from build123d import *

# Parameters (mm, degrees)
SKETCH2_R           = 1.5
BOSS_EXTRUDE1_DEPTH = 5


with BuildPart() as part:
    # Sketch2 → Boss-Extrude1 (new body)
    with BuildSketch(Plane.XY):
        with BuildLine():
            Line((2.043003371, 9.789082553), (85.846562924, -7.700907316))
            Line((85.846562924, -7.700907316), (81.760556182, -27.279072422))
            Line((81.760556182, -27.279072422), (-2.043003371, -9.789082553))
            ThreePointArc((-2.043003371, -9.789082553), (-9.789082553, 2.043003371), (2.043003371, 9.789082553))
        make_face()
        Circle(SKETCH2_R, mode=Mode.SUBTRACT)
        with Locations((0, 7)):
            Circle(SKETCH2_R, mode=Mode.SUBTRACT)
        with Locations((0, -7)):
            Circle(SKETCH2_R, mode=Mode.SUBTRACT)
        with Locations((7, 0)):
            Circle(SKETCH2_R, mode=Mode.SUBTRACT)
        with Locations((-7, 0)):
            Circle(SKETCH2_R, mode=Mode.SUBTRACT)
        Polygon((74.456281443, -8.470092426), (67.882907111, -10.632764358), (66.469148778, -17.406809485), (71.628764778, -22.018182679), (78.20213911, -19.855510747), (79.615897443, -13.08146562), align=None, mode=Mode.SUBTRACT)
    extrude(amount=BOSS_EXTRUDE1_DEPTH)


solid = part.part
Design review of the part built by this model. Coordinates are the model's own, in mm. A direction names the side the tool comes from. Round coordinates to 2 decimals unless told otherwise and drop trailing zeros. Loops run counter-clockwise (first coordinate to the right, second up) from the corner with the lowest first, then second, coordinate; pieces in that order, holes last. Notation, with made-up numbers: (88.25, -7) - (111.25, -7) arc R21 cw to (111.25, 17) - close; hole circle Ø10 at (-19.5, -17). An arc over 180 degrees is marked (long way). One line per item, written item: value. Start each with the question number.
1) Consider section A-A on z = 1.55. Give the boundary of the cut face in (x, y).
2) Draft analysis for pull direction Y (two halves, no side actions). For faces 3 (the cylindrical face through (-0.325, -8.464, 2.465)), 4 (the flat face through (43.358, 1.167, 2.465)), 5 (the flat face through (69.01, -19.68, 2.46)), 6 (the cylindrical face through (-9.83, 1.83, 2.46)), state which applies: +Y half, -Y half, draft (parallel to the pull), parting line (faces both ways), or undercut.
3) Consider section C-C on x = 73.5. Give the boundary of the cut face in (y, z).
4) To check wall thickness, follow L1, parallel to Y at x = 0, z = 3.9; L2, parallel to Y at x = 7, z = 2.15; L3, parallel to Y at x = 77.5, z = 1.5. State the ranges of each line that lie inside material, in increasing order. Write a range as from..to.
5) Consider section B-B on y = 0. Give the boundary of the cut face in (x, z).
6) Consider section D-D on y = -21. Give the boundary of the cut face in (x, z).
7) Insertion check: pin 1 Ø12 at (x, y) = (27, -11) entering from -Z; pin 2 Ø1.5 at (y, z) = (-15.5, 1) entering from +X; pin 3 Ø1.5 at (y, z) = (-10, 3) entering from -X; pin 4 Ø1 at (y, z) = (-17.5, 1.5) entering from +X. Each pin has a flat end and moves straight along its axis. Give the tip position at first contact, or say it passes through.
8) For faces 1 (the flat face through (67.186, -13.972, 2.465)), 2 (the flat face through (39, -8, 0)), list the 3-axis set-ups (+Z, -Z, +X, -X, +Y, -Y) from which the entire face can be reached by the end or side of a thin tool; tool diameter is ignored.
Reported:
1. outline: (-2.04, -9.79) - (81.76, -27.28) - (85.85, -7.7) - (2.04, 9.79) arc R10 ccw to start; hole circle Ø3 at (-7, 0); hole circle Ø3 at (0, -7); hole circle Ø3 at (0, 0); hole circle Ø3 at (0, 7); hole circle Ø3 at (7, 0); hole (66.47, -17.41) - (71.63, -22.02) - (78.2, -19.86) - (79.62, -13.08) - (74.46, -8.47) - (67.88, -10.63) - close
2. face 3: undercut
2. face 4: +Y half
2. face 5: undercut
2. face 6: parting line
3. outline: (-25.56, 0) - (-21.4, 0) - (-21.4, 5) - (-25.56, 5) - close; (-8.78, 0) - (-5.12, 0) - (-5.12, 5) - (-8.78, 5) - close
4. L1: y = -10.22..-8.5, -5.5..-1.5, 1.5..5.5, 8.5..10
4. L2: y = -11.68..-1.5, 1.5..8.75
4. L3: y = -26.39..-20.09, -11.19..-5.96
5. outline: (-10, 0) - (-8.5, 0) - (-8.5, 5) - (-10, 5) - close; (-5.5, 0) - (-1.5, 0) - (-1.5, 5) - (-5.5, 5) - close; (1.5, 0) - (5.5, 0) - (5.5, 5) - (1.5, 5) - close; (8.5, 0) - (48.95, 0) - (48.95, 5) - (8.5, 5) - close
6. outline: (51.67, 0) - (70.49, 0) - (70.49, 5) - (51.67, 5) - close; (74.72, 0) - (83.07, 0) - (83.07, 5) - (74.72, 5) - close
7. pin 1: stops at z = 0
7. pin 2: stops at x = 84.38
7. pin 3: stops at x = -3.8
7. pin 4: stops at x = 83.91
8. face 1: +Z, -Z
8. face 2: -Z, +X, -X, +Y, -Y
